Geometry: final body of the model. Coordinates: model frame, mm. A direction names the side the tool comes from. Coordinates: 2 decimals unless noted, no trailing zeros. Loops run counter-clockwise (first coordinate to the right, second up) from the corner with the lowest first, then second, coordinate; pieces in that order, holes last. Notation, with made-up numbers: (-30, 85.25) -> (-21, 85.25) arc R24 ccw to (-21, 117.25) -> close; hole circle Ø3 at (35, -33). An arc over 180 degrees is marked (long way). One line per item, written item: value. Start each with the question number.
from build123d import *

# Parameters (mm, degrees)
BOSS_EXTRUDE1_DEPTH = 11
CLEAR_HOLE_BOLT_R   = 3.7
CLEAR_HOLE_BOLT_R_2 = 2.6
CUT_EXTRUDE1_DEPTH  = 56.011362463
SKETCH5_R           = 3
SKETCH5_W           = 5
SKETCH5_H           = 15
BOSS_EXTRUDE2_DEPTH = 7
M3_SUPPORT_HOLES_R  = 1.6
CUT_EXTRUDE2_DEPTH  = 57.826490302
CUT_EXTRUDE4_DEPTH  = 3
SKETCH7_R           = 5.25
SKETCH7_R_2         = 6.375
BOSS_EXTRUDE3_DEPTH = 7
CUT_EXTRUDE5_START  = -32.5
CUT_EXTRUDE5_DEPTH  = 65
SKETCH24_R          = 1.6
CUT_EXTRUDE7_DEPTH  = 64.877232071
CUT_EXTRUDE8_START  = -15.5
CUT_EXTRUDE8_DEPTH  = 20
SKETCH26_W          = 3
SKETCH26_H          = 5
BOSS_EXTRUDE7_DEPTH = 5
SKETCH27_R          = 1.25
CUT_EXTRUDE9_DEPTH  = 3
FILLET1_R           = 2.5
FILLET2_R           = 2


# Read off the part's stored shape, not the designer's step: Cut-Extrude5, Boss-Extrude6
with BuildPart() as part:
    # Main Body → Boss-Extrude1 (new body)
    with BuildSketch(Plane(origin=(0, 0, 0), x_dir=(0, 0, -1), z_dir=(1, 0, 0))):
        with BuildLine():
            Line((-38, 32.5), (38, 32.5))
            ThreePointArc((38, 32.5), (41.535533906, 31.035533906), (43, 27.5))
            Line((43, 27.5), (43, -27.5))
            ThreePointArc((43, -27.5), (41.535533906, -31.035533906), (38, -32.5))
            Line((38, -32.5), (-38, -32.5))
            ThreePointArc((-38, -32.5), (-41.535533906, -31.035533906), (-43, -27.5))
            Line((-43, -27.5), (-43, 27.5))
            ThreePointArc((-43, 27.5), (-41.535533906, 31.035533906), (-38, 32.5))
        make_face()
    extrude(amount=BOSS_EXTRUDE1_DEPTH)

    # Clear Hole-Bolt → Cut-Extrude1 (cut, through all)
    with BuildSketch(Plane(origin=(11, 0, 0), x_dir=(0, 0, -1), z_dir=(1, 0, 0))):
        with Locations((29.85, 20)):
            Circle(CLEAR_HOLE_BOLT_R)
        with Locations((-29.85, 20)):
            Circle(CLEAR_HOLE_BOLT_R_2)
        with Locations(Location((-29.85, -20, 0), (0, 0, 180))):
            Circle(CLEAR_HOLE_BOLT_R_2)
        with Locations(Location((29.85, -20, 0), (0, 0, 180))):
            Circle(CLEAR_HOLE_BOLT_R)
    extrude(amount=-CUT_EXTRUDE1_DEPTH, mode=Mode.SUBTRACT)

    # Sketch5 → Boss-Extrude2 (add)
    with BuildSketch(Plane(origin=(11, 0, 0), x_dir=(0, 0, -1), z_dir=(1, 0, 0))):
        with Locations((10.35, -7.5)):
            Circle(SKETCH5_R)
        with Locations(Location((10.35, 7.5, 0), (0, 0, 180))):
            Circle(SKETCH5_R)
        with Locations((11.3, -25)):
            Rectangle(SKETCH5_W, SKETCH5_H)
        with Locations((3.4, -25)):
            Rectangle(SKETCH5_W, SKETCH5_H)
        with Locations((11.3, 25)):
            Rectangle(SKETCH5_W, SKETCH5_H)
        with Locations((3.4, 25)):
            Rectangle(SKETCH5_W, SKETCH5_H)
    extrude(amount=BOSS_EXTRUDE2_DEPTH)

    # M3 Support Holes → Cut-Extrude2 (cut, through all)
    with BuildSketch(Plane(origin=(18, 0, 0), x_dir=(0, 0, -1), z_dir=(1, 0, 0))):
        with Locations((10.35, 7.5)):
            Circle(M3_SUPPORT_HOLES_R)
        with Locations(Location((10.35, -7.5, 0), (0, 0, 180))):
            Circle(M3_SUPPORT_HOLES_R)
    extrude(amount=-CUT_EXTRUDE2_DEPTH, mode=Mode.SUBTRACT)

    # M3 Nut Support → Cut-Extrude4 (cut)
    with BuildSketch(Plane.ZY):
        Polygon((-8.617949192, 10.5), (-12.082050808, 10.5), (-13.814101615, 7.5), (-12.082050808, 4.5), (-8.617949192, 4.5), (-6.885898385, 7.5), align=None)
        Polygon((-6.885898385, -7.5), (-8.617949192, -10.5), (-12.082050808, -10.5), (-13.814101615, -7.5), (-12.082050808, -4.5), (-8.617949192, -4.5), align=None)
    extrude(amount=-CUT_EXTRUDE4_DEPTH, mode=Mode.SUBTRACT)

    # Sketch7 → Boss-Extrude3 (add)
    # profile 1 of 2: a face of its own
    with BuildSketch(Plane(origin=(11, 0, 0), x_dir=(0, 0, -1), z_dir=(1, 0, 0))):
        with BuildLine():
            Line((5.9, 32.5), (5.9, -32.5))
            Line((5.9, -32.5), (-38, -32.5))
            ThreePointArc((-38, -32.5), (-41.535533906, -31.035533906), (-43, -27.5))
            Line((-43, -27.5), (-43, 27.5))
            ThreePointArc((-43, 27.5), (-41.535533906, 31.035533906), (-38, 32.5))
            Line((-38, 32.5), (5.9, 32.5))
        make_face()
        with Locations((-29.85, -20)):
            Circle(SKETCH7_R, mode=Mode.SUBTRACT)
        with Locations(Location((-29.85, 20, 0), (0, 0, 180))):
            Circle(SKETCH7_R, mode=Mode.SUBTRACT)
    # profile 2 of 2: a face of its own
    with BuildSketch(Plane(origin=(11, 0, 0), x_dir=(0, 0, -1), z_dir=(1, 0, 0))):
        with BuildLine():
            Line((13.8, 32.5), (13.8, 17.5))
            Line((13.8, 17.5), (14.05, 17.5))
            ThreePointArc((14.05, 17.5), (16.701650429, 16.401650429), (17.8, 13.75))
            Line((17.8, 13.75), (17.8, -13.75))
            ThreePointArc((17.8, -13.75), (16.701650429, -16.401650429), (14.05, -17.5))
            Line((14.05, -17.5), (13.8, -17.5))
            Line((13.8, -17.5), (13.8, -32.5))
            Line((13.8, -32.5), (38, -32.5))
            ThreePointArc((38, -32.5), (41.535533906, -31.035533906), (43, -27.5))
            Line((43, -27.5), (43, 27.5))
            ThreePointArc((43, 27.5), (41.535533906, 31.035533906), (38, 32.5))
            Line((38, 32.5), (13.8, 32.5))
        make_face()
        with Locations((29.85, -20)):
            Circle(SKETCH7_R_2, mode=Mode.SUBTRACT)
        with Locations(Location((29.85, 20, 0), (0, 0, 180))):
            Circle(SKETCH7_R_2, mode=Mode.SUBTRACT)
    extrude(amount=BOSS_EXTRUDE3_DEPTH)

    # Cut-Extrude5 outline → Cut-Extrude5 (cut)
    with BuildSketch(Plane(origin=(0, 0, 0), x_dir=(1, 0, 0), z_dir=(0, 1, 0)).offset(CUT_EXTRUDE5_START)):
        Polygon((18, -10.348779336), (18, -4.351220664), (9.5, -5.85), (9.5, -8.85), align=None)
    extrude(amount=CUT_EXTRUDE5_DEPTH, mode=Mode.SUBTRACT)

    # Boss-Extrude6 outline → Boss-Extrude6 (revolve)
    with BuildSketch(Plane(origin=(5.019399377, 5.981887241, 25), x_dir=(0.6427876096865357, 0.7660444431189811, 0), z_dir=(0, 0, -1))):
        Polygon((5.590261427, 12.222600941), (2.75, 19.252494658), (0, 19.252494658), (0, 12.222600941), align=None)
    boss_extrude6 = revolve(axis=Axis((5.019399377, 5.981887241, 25), (0.7660444431189813, -0.6427876096865358, 0)))

    # Sketch24 → Cut-Extrude7 (cut, through all)
    with BuildSketch(Plane(origin=(14.748266549, -12.375265022, 0), x_dir=(0, 0, -1), z_dir=(0.7660444431189812, -0.6427876096865357, 0))):
        with Locations(Location((-25, 7.808799208, 0), (0, 0, 90))):
            Circle(SKETCH24_R)
    cut_extrude7 = extrude(amount=-CUT_EXTRUDE7_DEPTH, mode=Mode.SUBTRACT)

    # Sketch25 → Cut-Extrude8 (cut)
    with BuildSketch(Plane(origin=(14.748266549, -12.375265022, 0), x_dir=(0, 0, -1), z_dir=(0.7660444431189812, -0.6427876096865356, 0)).offset(CUT_EXTRUDE8_START)):
        Polygon((-23.267949192, 10.808799208), (-26.732050808, 10.808799208), (-28.464101615, 7.808799208), (-26.732050808, 4.808799208), (-23.267949192, 4.808799208), (-21.535898385, 7.808799208), align=None)
    cut_extrude8 = extrude(amount=-CUT_EXTRUDE8_DEPTH, mode=Mode.SUBTRACT)

    # Mirror2: Boss-Extrude6, Cut-Extrude7, Cut-Extrude8 across plane
    add(boss_extrude6.mirror(Plane.XY))
    add(cut_extrude7.mirror(Plane.XY), mode=Mode.SUBTRACT)
    add(cut_extrude8.mirror(Plane.XY), mode=Mode.SUBTRACT)

    # Sketch26 → Boss-Extrude7 (add)
    with BuildSketch(Plane(origin=(18, 0, 0), x_dir=(0, 0, -1), z_dir=(1, 0, 0))):
        with Locations((0, -11)):
            Rectangle(SKETCH26_W, SKETCH26_H)
    extrude(amount=BOSS_EXTRUDE7_DEPTH)

    # Sketch27 → Cut-Extrude9 (cut)
    with BuildSketch(Plane.XY.offset(1.5)):
        with Locations((20.5, -11)):
            Circle(SKETCH27_R)
    extrude(amount=-CUT_EXTRUDE9_DEPTH, mode=Mode.SUBTRACT)

    # Fillet1
    fillet1_edges = [part.edges().sort_by_distance(p)[0] for p in [
        (23, -13.5, 0),
        (23, -8.5, 0),
    ]]
    fillet(fillet1_edges, radius=FILLET1_R - 0.0001)  # a hair under: the kernel refuses the full size

    # Fillet2
    fillet2_edges = [part.edges().sort_by_distance(p)[0] for p in [
        (18, -8.5, 0),
        (18, -13.5, 0),
    ]]
    fillet(fillet2_edges, radius=FILLET2_R)


solid = part.part
1. Line query: L1, parallel to Y at x = 5.75, z = 29.85; L2, parallel to Z at x = 2.5, y = -20; L3, parallel to Y at x = 10.5, z = -10.35. Output: solid intervals per line, ascending. Write a range as [from, to].
2. Set-up query: faces 1 (the face through (8.778, 4.623, 23.509)), 2 (the face through (14.45, 22.01, 34.7)), 3 (the face through (1.48, -6.02, -12.96)), 4 (the face through (14, 0, -5.9)). Return all of +Z, -Z, +X, -X, +Y, -Y with unobstructed straight access to the full face (end or side cutting, diameter ignored); none if empty.
3. Section B-B on z = -10.35. Count the separate pieces of the cut face and the enclosed holes in it, plus the area to 3 significant figures.
4. Pin query (flat end, axial travel): pin 1 Ø10 at (y, z) = (-19.5, -30) entering from +X; pin 2 Ø5 at (y, z) = (-8.5, -10.5) entering from +X; pin 3 Ø1.8 at (y, z) = (6.5, -10.5) entering from -X; pin 4 Ø10 at (x, z) = (20.5, -17) entering from +Y. Return the tip coordinate at first contact, or that it passes through.
5. Section C-C on z = 29.85. Return the cut outline in (x, y), plus the area to 3 significant figures.
6. Section A-A on y = -20. Return the cut outline in (x, z) (3 decimals).
7. Draft query along Z for faces 5 (the face through (20.92, -5.02, 25.04)), 6 (the face through (9, 0, -43)), 7 (the face through (9, 0, 43)), 8 (the face through (14.45, -5.47, -8.14)). Return one class per face: released by +Z, released by -Z, zero draft, split by the parting line, or undercut.
Checks:
1. L1: [-32.5, -22.6], [-17.4, 17.4], [22.6, 32.5]
1. L2: [-43, -33.55], [-26.15, 27.25], [32.45, 43]
1. L3: [-32.5, -9.1], [-5.9, 5.9], [9.1, 32.5]
2. face 1: none
2. face 2: +X
2. face 3: -X
2. face 4: +X, +Y, -Y
3. separate pieces: 3
3. enclosed holes: 0
3. area: 877 mm²
4. pin 1: x = 11
4. pin 2: x = 18
4. pin 3: x = 3
4. pin 4: y = 32.5
5. outline: (0, -32.5) -> (18, -32.5) -> (18, -25.25) -> (11, -25.25) -> (11, -22.6) -> (0, -22.6) -> close; (0, -17.4) -> (11, -17.4) -> (11, -14.75) -> (18, -14.75) -> (18, 14.75) -> (11, 14.75) -> (11, 17.4) -> (0, 17.4) -> close; (0, 22.6) -> (11, 22.6) -> (11, 25.25) -> (18, 25.25) -> (18, 32.5) -> (0, 32.5) -> close
5. area: 909 mm²
6. outline: (0, -43) -> (18, -43) -> (18, -36.225) -> (11, -36.225) -> (11, -33.55) -> (0, -33.55) -> close; (0, -26.15) -> (11, -26.15) -> (11, -23.475) -> (18, -23.475) -> (18, -8.8) -> (11, -8.8) -> (11, -5.9) -> (18, -5.9) -> (18, 4.351) -> (9.5, 5.85) -> (9.5, 8.85) -> (18, 10.349) -> (18, 24.6) -> (11, 24.6) -> (11, 27.25) -> (0, 27.25) -> close; (0, 32.45) -> (11, 32.45) -> (11, 35.1) -> (18, 35.1) -> (18, 43) -> (0, 43) -> close
7. face 5: zero draft
7. face 6: released by -Z
7. face 7: released by +Z
7. face 8: undercut
